Check sheet for the modelled part. Datum: model origin and axes. Units: mm. A direction names the side the tool comes from. Round coordinates to 2 decimals unless told otherwise and drop trailing zeros. Order: outer loops, then holes, each group sorted by start corner. A loop starts at its lowest first (then second) coordinate and runs counter-clockwise, first axis right, second up.
Q1. Cross-section at B-B on y = -102. Record the cut outline in (x, z).
Q2. Cross-section at D-D on y = 264.5. Record the cut outline in (x, z), then the cut area to 3 significant figures.
Q3. Mould release check, pull along Y, two halves, no side actions. Record for faces 4 (the cylindrical face through (-72.63, -383.75, -13.75)), 5 (the cylindrical face through (-72.63, 383.75, -13.74)), 6 (the flat face through (1.422, 269.171, 3.135)): +Y half, -Y half, draft (parallel to the pull), parting line (faces both ways), or undercut.
Q4. Scan lines: probe 1 along Z at (x, y) = (66.5, 319); probe 2 along Z at (x, y) = (91, 77.5). Record each from-to range of solid material in increasing order.
Q5. Set-up check for faces 1 (the flat face through (-1, 3, 0.794)), 2 (the flat face through (-1, 3, 0)), 3 (the flat face through (1.422, 346.256, -5.014)): record each of +Z, -Z, +X, -X, +Y, -Y from which the full face is reachable in a straight line by a thin tool's end or side.
Q6. Cross-section at C-C on x = -81. Record the cut outline in (y, z).
Q7. Depth check by flat-ended pin: P1, Ø10, axis at x = -79, z = -16.5, coming from the +Y side; P2, Ø8, axis at x = -68.5, y = 109, coming from the +Z side; P3, Ø1, axis at x = 16.5, y = -204.5, coming from the -Z side. Enter the tip coordinate at first touch or a pass-through.
Q8. Cross-section at A-A on x = -40. Record the cut outline in (y, z), then the cut area to 3 significant figures.
from build123d import *

# Parameters (mm, degrees)
F0_W     = 203.2
F0_H     = 482.6
F1_DEPTH = 0.79375
F3_DEPTH = 203.2
F4_R     = 101.59999


# Not quite as in the source:
# - a fillet or chamfer is up to 0.001 mm smaller than in the source, because OpenCascade refuses the exact size


with BuildPart() as f1:
    # F0 (on Top) → F1 (new body)
    with BuildSketch(Plane.XY):
        Rectangle(F0_W, F0_H)
    extrude(amount=F1_DEPTH)

    # F2 (on face) → F3 (join, through all)
    with BuildSketch(Plane.YZ.offset(101.6)):
        with BuildLine():
            ThreePointArc((243.5137558658, 0.8904046685), (242.4079324391, 0.8179251718), (241.3, 0.79375))
            Line((241.3, 0.79375), (241.3, 0))
            ThreePointArc((241.3, 0), (242.4425553278, 0.0249306459), (243.5829357366, 0.0996751269))
            Line((243.5829357366, 0.0996751269), (294.1896263997, 4.5271868584))
            ThreePointArc((294.1896263997, 4.5271868584), (298.0689507117, 4.5691740706), (301.9094190229, 4.0198807111))
            Line((301.9094190229, 4.0198807111), (413.4915953519, -20.7572846976))
            Line((413.4915953519, -20.7572846976), (413.6636590006, -19.9824084731))
            Line((413.6636590006, -19.9824084731), (302.0814826716, 4.7947569356))
            ThreePointArc((302.0814826716, 4.7947569356), (298.1209997257, 5.3612157126), (294.1204465289, 5.3179164001))
            Line((294.1204465289, 5.3179164001), (243.5137558658, 0.8904046685))
        make_face()
        with BuildLine():
            Line((-241.3, 0), (-241.3, 0.79375))
            ThreePointArc((-241.3, 0.79375), (-242.4079324391, 0.8179251718), (-243.5137558658, 0.8904046685))
            Line((-243.5137558658, 0.8904046685), (-294.1204465289, 5.3179164001))
            ThreePointArc((-294.1204465289, 5.3179164001), (-298.1209997257, 5.3612157126), (-302.0814826716, 4.7947569356))
            Line((-302.0814826716, 4.7947569356), (-413.6636590006, -19.9824084731))
            Line((-413.6636590006, -19.9824084731), (-413.4915953519, -20.7572846976))
            Line((-413.4915953519, -20.7572846976), (-301.9094190229, 4.0198807111))
            ThreePointArc((-301.9094190229, 4.0198807111), (-298.0689507117, 4.5691740706), (-294.1896263997, 4.5271868584))
            Line((-294.1896263997, 4.5271868584), (-243.5829357366, 0.0996751269))
            ThreePointArc((-243.5829357366, 0.0996751269), (-242.4425553278, 0.0249306459), (-241.3, 0))
        make_face()
    extrude(amount=-F3_DEPTH)

    # F4 (radius 101.6 in the source; OpenCascade refuses exactly that, so slightly less here)
    f4_edges = [f1.edges().sort_by_distance(p)[0] for p in [
        (101.6, 413.577627, -20.369847),
        (-101.6, 413.577627, -20.369847),
        (101.6, -413.577627, -20.369847),
        (-101.6, -413.577627, -20.369847),
    ]]
    fillet(f4_edges, radius=F4_R)


solid = f1.part
Results found:
1. outline: (-101.6, 0) - (101.6, 0) - (101.6, 0.79) - (-101.6, 0.79) - close
2. outline: (-101.6, 1.93) - (101.6, 1.93) - (101.6, 2.73) - (-101.6, 2.73) - close
2. area: 162 mm2
3. face 4: -Y half
3. face 5: +Y half
3. face 6: undercut
4. probe 1: z = 0.22 to 1.04
4. probe 2: z = 0 to 0.79
5. face 1: +Z, +X, -X
5. face 2: -Z, +X, -X
5. face 3: +Z, +X, -X, +Y
6. outline: (-374.35, -11.25) - (-374.18, -12.03) - (-301.91, 4.02) arc R25.4 cw to (-294.19, 4.53) - (-243.58, 0.1) arc R26.19 ccw to (-241.3, 0) - (241.3, 0) arc R26.19 ccw to (243.58, 0.1) - (294.19, 4.53) arc R25.4 cw to (301.91, 4.02) - (374.18, -12.03) - (374.35, -11.25) - (302.08, 4.79) arc R26.19 ccw to (294.12, 5.32) - (243.51, 0.89) arc R25.4 cw to (241.3, 0.79) - (-241.3, 0.79) arc R25.4 cw to (-243.51, 0.89) - (-294.12, 5.32) arc R26.19 ccw to (-302.08, 4.79) - close
7. P1: stops at y = 381.3
7. P2: stops at z = 0.79
7. P3: stops at z = 0
8. outline: (-405.65, -18.2) - (-405.48, -18.98) - (-301.91, 4.02) arc R25.4 cw to (-294.19, 4.53) - (-243.58, 0.1) arc R26.19 ccw to (-241.3, 0) - (241.3, 0) arc R26.19 ccw to (243.58, 0.1) - (294.19, 4.53) arc R25.4 cw to (301.91, 4.02) - (405.48, -18.98) - (405.65, -18.2) - (302.08, 4.79) arc R26.19 ccw to (294.12, 5.32) - (243.51, 0.89) arc R25.4 cw to (241.3, 0.79) - (-241.3, 0.79) arc R25.4 cw to (-243.51, 0.89) - (-294.12, 5.32) arc R26.19 ccw to (-302.08, 4.79) - close
8. area: 648 mm2
